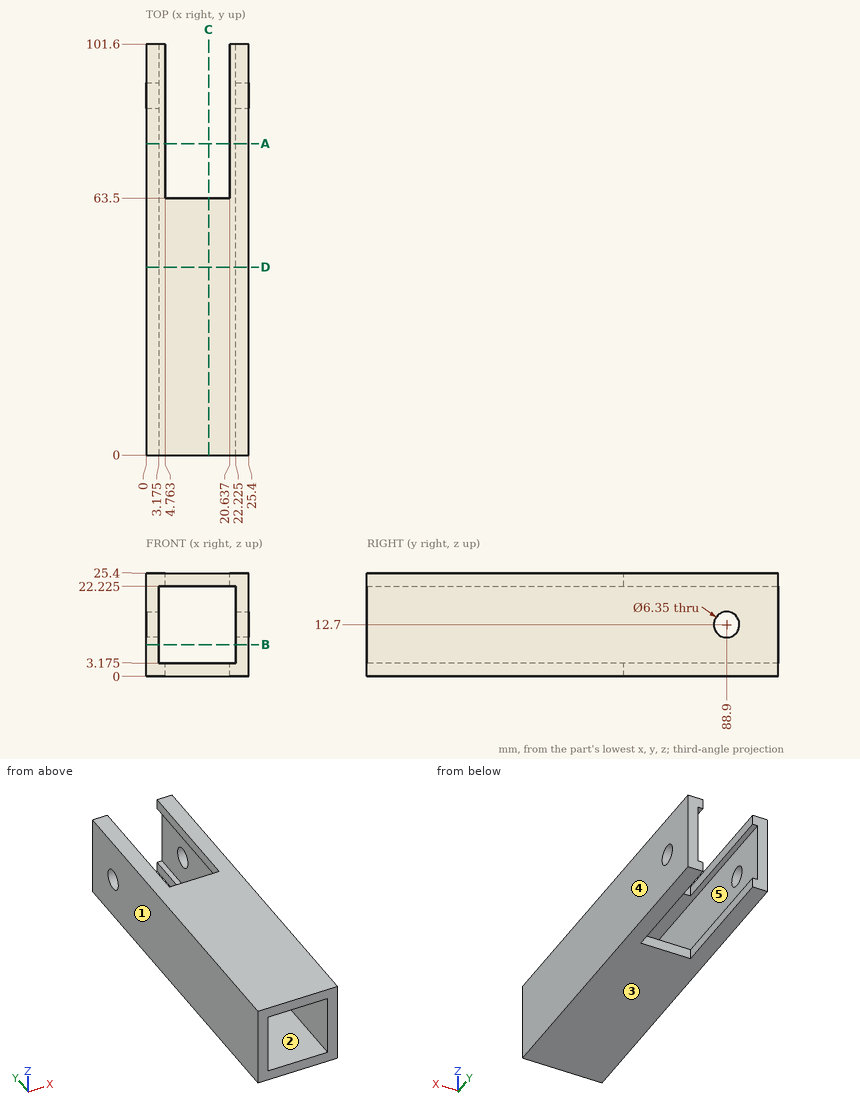
Study the drawing (mm; zero at the part's minimum x, y, z) and answer. A direction names the side the tool comes from. Give positions to 0.01 mm unless a question says otherwise; leave off trailing zeros. Write each loop counter-clockwise with the first axis right and the second up, starting at its lowest first coordinate (ties: lowest second). Pieces come first, ordered by that corner, then holes. Notation, with made-up numbers: (24.25, 10) - (28.25, 10) arc R23 cw to (28.25, 32) - close; hole circle Ø5 at (-30.75, -5.5). An arc over 180 degrees is marked (long way). Write item = value, one per line. Start each with the question number.
Item 1: Find the intervals of material crossed by probe 1 along Z at (x, y) = (22, 22) (1 decimal); probe 2 along Y at (x, z) = (1.35, 12.7) (1 decimal), in increasing order. Write a range as [from, to].
Item 2: Find section D-D (y = 46.5). Give the vertices of the cut face in (x, z) (1 decimal).
Item 3: Find section C-C (x = 15.5). Give the vertices of the cut face in (y, z) (1 decimal), then the cut area to 3 significant figures.
Item 4: This flat-tipped pin is pushed along its axis until it touches: P1, Ø3.5, axis at x = 10.5, z = 2, coming from the +Y side. Where does it stop, or does it pass through?
Item 5: Find section A-A (y = 77). Give the vertices of the cut face in (x, z) (1 decimal).
Item 6: The mould has two halves that part along Z. Classify the marked faces 3, 4 and 5: +Z half, -Z half, draft (parallel to the pull), parting line (faces both ways), or undercut.
Item 7: A tool of negligible diameter and unlimited length cuts with its end or side. For the marked faces 1 and 2, from which of +Z, -Z, +X, -X, +Y, -Y can it reach the whole face along a straight path? Write none if from no direction.
Item 8: Find section B-B (z = 7.75). Give the vertices of the cut face in (x, y) (1 decimal).
Response:
q1.probe_1 = [0, 3.2], [22.2, 25.4]
q1.probe_2 = [0, 85.7], [92.1, 101.6]
q2.outline = (0, 0) - (25.4, 0) - (25.4, 25.4) - (0, 25.4) - close; hole (3.2, 3.2) - (22.2, 3.2) - (22.2, 22.2) - (3.2, 22.2) - close
q3.outline = (0, 0) - (63.5, 0) - (63.5, 3.2) - (0, 3.2) - close; (0, 22.2) - (63.5, 22.2) - (63.5, 25.4) - (0, 25.4) - close
q3.area = 403 mm²
q4.P1 = 63.5
q5.outline = (0, 0) - (4.8, 0) - (4.8, 3.2) - (3.2, 3.2) - (3.2, 22.2) - (4.8, 22.2) - (4.8, 25.4) - (0, 25.4) - close; (20.6, 0) - (25.4, 0) - (25.4, 25.4) - (20.6, 25.4) - (20.6, 22.2) - (22.2, 22.2) - (22.2, 3.2) - (20.6, 3.2) - close
q6.face_3 = -Z half
q6.face_4 = draft
q6.face_5 = undercut
q7.face_1 = +Z, -Z, -X, +Y, -Y
q7.face_2 = +Y, -Y
q8.outline = (0, 0) - (3.2, 0) - (3.2, 101.6) - (0, 101.6) - close; (22.2, 0) - (25.4, 0) - (25.4, 101.6) - (22.2, 101.6) - close
